```python
from build123d import *

# Parameters (mm, degrees)
ESTRUSIONE_ESTRUSIONE1_OUTLINE_W   = 10
ESTRUSIONE_ESTRUSIONE1_OUTLINE_H   = 10
ESTRUSIONE_ESTRUSIONE1_OUTLINE_W_2 = 8
ESTRUSIONE_ESTRUSIONE1_OUTLINE_H_2 = 3
ESTRUSIONE_ESTRUSIONE1_OUTLINE_W_3 = 12
ESTRUSIONE_ESTRUSIONE1_OUTLINE_H_3 = 22.6
ESTRUSIONE_ESTRUSIONE1_DEPTH       = 4
RACCORDO1_R                        = 1
RACCORDO3_R                        = 1
RACCORDO4_R                        = 0.3


# Read off the part's stored shape, not the designer's step: Estrusione-Estrusione1
with BuildPart() as part:
    # Estrusione-Estrusione1 outline → Estrusione-Estrusione1 (new body)
    with BuildSketch(Plane.XY):
        with BuildLine():
            add(Edge.make_bspline(
                [(39.5, 29.6), (43.506938427, 25.593061573), (43.493061573, 14.8), (43.506938427, 4.006938427), (39.5, 0)],
                knots=[0, 0, 0, 0, 0.5, 1, 1, 1, 1], degree=3))
            Line((39.5, 29.6), (39.5, 26.1))
            Line((39.5, 26.1), (35.5, 26.1))
            Line((35.5, 26.1), (35.5, 29.6))
            add(Edge.make_bspline(
                [(35.5, 29.6), (31.962623794, 26.062612753), (26.4060962, 25.659880805), (20.342579531, 28.112334068), (15.848598331, 29.600000017)],
                knots=[0, 0, 0, 0, 0.358970883, 0.890087037, 0.890087037, 0.890087037, 0.890087037], degree=3))
            Line((15.848598331, 29.600000017), (15.7, 29.6))
            ThreePointArc((15.7, 29.6), (0, 32.400991179), (-15.7, 29.6))
            Line((-15.7, 29.6), (-15.848598331, 29.600000017))
            add(Edge.make_bspline(
                [(-35.5, 29.6), (-31.962623794, 26.062612753), (-26.4060962, 25.659880805), (-20.342579531, 28.112334068), (-15.848598331, 29.600000017)],
                knots=[0, 0, 0, 0, 0.358970883, 0.890087037, 0.890087037, 0.890087037, 0.890087037], degree=3))
            Line((-35.5, 29.6), (-35.5, 26.1))
            Line((-35.5, 26.1), (-39.5, 26.1))
            Line((-39.5, 26.1), (-39.5, 29.6))
            add(Edge.make_bspline(
                [(-39.5, 29.6), (-43.506938427, 25.593061573), (-43.493061573, 14.8), (-43.506938427, 4.006938427), (-39.5, 0)],
                knots=[0, 0, 0, 0, 0.5, 1, 1, 1, 1], degree=3))
            Line((-39.5, 0), (-39.5, 3.5))
            Line((-39.5, 3.5), (-35.5, 3.5))
            Line((-35.5, 3.5), (-35.5, 0))
            add(Edge.make_bspline(
                [(-35.5, 0), (-24.124671667, -0.699725618), (-28.237292398, 1.331108434), (-12.322535381, -4.786451171)],
                knots=[0, 0, 0, 0, 1, 1, 1, 1], degree=3))
            ThreePointArc((-12.322535381, -4.786451171), (0, -6.987919299), (12.322535381, -4.786451171))
            add(Edge.make_bspline(
                [(35.5, 0), (24.124671667, -0.699725618), (28.237292398, 1.331108434), (12.322535381, -4.786451171)],
                knots=[0, 0, 0, 0, 1, 1, 1, 1], degree=3))
            Line((35.5, 0), (35.5, 3.5))
            Line((35.5, 3.5), (39.5, 3.5))
            Line((39.5, 3.5), (39.5, 0))
        make_face()
        with Locations((-17, 6.6)):
            Rectangle(ESTRUSIONE_ESTRUSIONE1_OUTLINE_W, ESTRUSIONE_ESTRUSIONE1_OUTLINE_H, mode=Mode.SUBTRACT)
        with Locations((0, -2.5)):
            Rectangle(ESTRUSIONE_ESTRUSIONE1_OUTLINE_W_2, ESTRUSIONE_ESTRUSIONE1_OUTLINE_H_2, mode=Mode.SUBTRACT)
        with Locations((17, 6.6)):
            Rectangle(ESTRUSIONE_ESTRUSIONE1_OUTLINE_W, ESTRUSIONE_ESTRUSIONE1_OUTLINE_H, mode=Mode.SUBTRACT)
        Polygon((-24.868240888, 23.524038765), (-15.020163358, 25.260520542), (-14.15192247, 20.336481777), (-24, 18.6), align=None, mode=Mode.SUBTRACT)
        with Locations((0, 16.3)):
            Rectangle(ESTRUSIONE_ESTRUSIONE1_OUTLINE_W_3, ESTRUSIONE_ESTRUSIONE1_OUTLINE_H_3, mode=Mode.SUBTRACT)
        Polygon((15.020163358, 25.260520542), (24.868240888, 23.524038765), (24, 18.6), (14.15192247, 20.336481777), align=None, mode=Mode.SUBTRACT)
    extrude(amount=ESTRUSIONE_ESTRUSIONE1_DEPTH)

    # Raccordo1
    raccordo1_edges = [part.edges().sort_by_distance(p)[0] for p in [
        (15.020163358, 25.260520542, 2),
        (14.15192247, 20.336481777, 2),
        (24, 18.6, 2),
        (24.868240888, 23.524038765, 2),
        (-24.868240888, 23.524038765, 2),
        (-24, 18.6, 2),
        (-14.15192247, 20.336481777, 2),
        (-15.020163358, 25.260520542, 2),
    ]]
    fillet(raccordo1_edges, radius=RACCORDO1_R)

    # Raccordo3
    raccordo3_edges = [part.edges().sort_by_distance(p)[0] for p in [
        (12, 11.6, 2),
        (12, 1.6, 2),
        (22, 1.6, 2),
        (22, 11.6, 2),
        (-22, 11.6, 2),
        (-22, 1.6, 2),
        (-12, 1.6, 2),
        (-12, 11.6, 2),
    ]]
    fillet(raccordo3_edges, radius=RACCORDO3_R)

    # Raccordo4
    raccordo4_edges = [part.edges().sort_by_distance(p)[0] for p in [
        (-35.5, 0, 2),
        (-39.5, 0, 2),
        (35.5, 0, 2),
        (39.5, 0, 2),
        (39.5, 29.6, 2),
        (35.5, 29.6, 2),
        (-39.5, 29.6, 2),
        (-35.5, 29.6, 2),
    ]]
    fillet(raccordo4_edges, radius=RACCORDO4_R)


solid = part.part
```
Can you work these out from the model? Positions are in its coordinate system, mm. A direction names the side the tool comes from. Round coordinates to 2 decimals unless told otherwise and drop trailing zeros. Loops run counter-clockwise (first coordinate to the right, second up) from the corner with the lowest first, then second, coordinate; pieces in that order, holes last.
Item 1: Which directions (+Z, -Z, +X, -X, +Y, -Y) give clear straight access to the entire face, cutting with the end or side of a thin tool? Please do faces 1 (the flat face through (1, 4, 4)), 2 (the flat face through (-37, 26.1, 2)), 3 (the flat face through (35.5, 2, 2)), 4 (the flat face through (6, 16, 2)).
Item 2: Suppose I cut it at B-B, the plane z = 0.75. State how many separate pieces and enclosed holes the cut face has, then the cut area to 3 significant figures.
Item 3: If we mould it in two halves opening along Y, with no side actions, what happens to faces 5 (the flat face through (-22, 7, 2)), 6 (the flat face through (38, 26.1, 2)), 7 (the flat face through (-35.5, 2, 2))? For each: +Y half, -Y half, draft (parallel to the pull), parting line (faces both ways), or undercut.
Item 4: Will these pins go through, and if not, where does the flat tip stop? pin 1 Ø2 at (x, z) = (-18, 3) entering from -Y; pin 2 Ø2 at (y, z) = (27, 2) entering from -X; pin 3 Ø2 at (y, z) = (2.5, 2) entering from +X.
Item 5: Suppose I cut it at C-C, the plane x = -8.5. Write out the boundary of the cut face in (y, z), then the cut area to 3 significant figures.
Item 6: Suppose I cut it at A-A, the plane x = 2.5. Write out the boundary of the cut face in (y, z).
Item 7: Please list where these lines run through material, in increasing order: L1, parallel to Y at x = 0, z = 0.3; L2, parallel to Y at x = -20.5, z = 0.9; L3, parallel to X at y = 6.5, z = 2.35.
Reported:
1. face 1: +Z, +X, -X, +Y, -Y
1. face 2: +Z, -Z, +Y
1. face 3: +Z, -Z, -Y
1. face 4: +Z, -Z
2. separate pieces: 1
2. enclosed holes: 6
2. area: 2,070 mm2
3. face 5: undercut
3. face 6: +Y half
3. face 7: draft
4. pin 1: stops at y = -3.01
4. pin 2: stops at x = -41.98
4. pin 3: stops at x = 41.94
5. outline: (-5.96, 0) - (31.6, 0) - (31.6, 4) - (-5.96, 4) - close
5. area: 150 mm2
6. outline: (-6.9, 0) - (-4, 0) - (-4, 4) - (-6.9, 4) - close; (-1, 0) - (5, 0) - (5, 4) - (-1, 4) - close; (27.6, 0) - (32.33, 0) - (32.33, 4) - (27.6, 4) - close
7. L1: y = -6.99 to -4, -1 to 5, 27.6 to 32.4
7. L2: y = -1.75 to 1.6, 11.6 to 19.22, 24.29 to 28.01
7. L3: x = -42.92 to -22, -12 to -6, 6 to 12, 22 to 42.92
